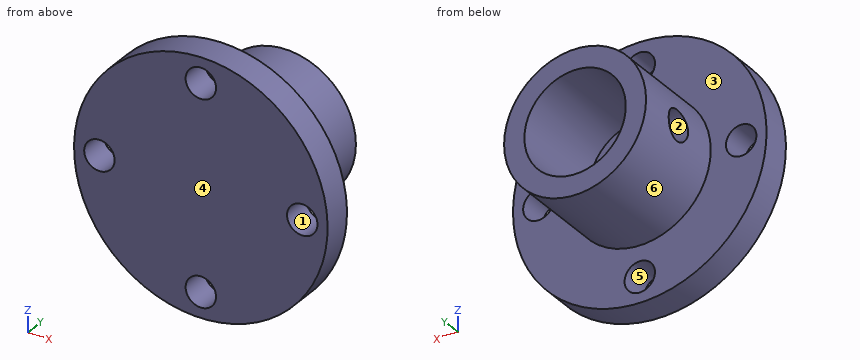
from build123d import *

# Parameters (mm, degrees)
IZIM1_R                     = 12.5
IZIM1_R_2                   = 1.5
Y_KSEKLIK_EKSTR_ZYON1_DEPTH = 3
IZIM2_R                     = 7
IZIM2_R_2                   = 5
EKSTR_ZYON_NCE1_DEPTH       = 10
IZIM3_R                     = 1.5
KES_EKSTR_ZYON1_DEPTH       = 22.943108257


with BuildPart() as part:
    # Çizim1 → Yükseklik-Ekstrüzyon1 (new body)
    with BuildSketch(Plane(origin=(0, 0, 0), x_dir=(1, 0, 0), z_dir=(0, 1, 0))):
        with Locations(Location((0, 0, 0), (0, 0, 270))):
            Circle(IZIM1_R)
        with Locations(Location((10, 0, 0), (0, 0, 270))):
            Circle(IZIM1_R_2, mode=Mode.SUBTRACT)
        with Locations(Location((0, -10, 0), (0, 0, 270))):
            Circle(IZIM1_R_2, mode=Mode.SUBTRACT)
        with Locations(Location((-10, 0, 0), (0, 0, 270))):
            Circle(IZIM1_R_2, mode=Mode.SUBTRACT)
        with Locations(Location((0, 10, 0), (0, 0, 270))):
            Circle(IZIM1_R_2, mode=Mode.SUBTRACT)
    extrude(amount=Y_KSEKLIK_EKSTR_ZYON1_DEPTH)

    # Çizim2 → Ekstrüzyon-İnce1 (add)
    with BuildSketch(Plane(origin=(0, 3, 0), x_dir=(1, 0, 0), z_dir=(0, 1, 0))):
        Circle(IZIM2_R)
        Circle(IZIM2_R_2, mode=Mode.SUBTRACT)
    extrude(amount=EKSTR_ZYON_NCE1_DEPTH)

    # Çizim3 → Kes-Ekstrüzyon1 (cut, through all)
    with BuildSketch(Plane(origin=(0, 0, 0), x_dir=(0, 0, -1), z_dir=(1, 0, 0))):
        with Locations((0, 8)):
            Circle(IZIM3_R)
    extrude(amount=-KES_EKSTR_ZYON1_DEPTH, mode=Mode.SUBTRACT)


solid = part.part
The listing builds one solid part. Answer for the finished solid, in the listing's coordinates (mm). Face numbers are marked on the shaded views. A direction names the side the tool comes from. Round coordinates to 2 decimals unless told otherwise and drop trailing zeros. Write each loop counter-clockwise with the first axis right and the second up, starting at its lowest first coordinate (ties: lowest second). Pieces come first, ordered by that corner, then holes. Notation, with made-up numbers: (-33, -1) - (-5, -1) arc R14 ccw to (-5, 23) - close; hole circle Ø6 at (11, 14). An arc over 180 degrees is marked (long way). Use one line per item in the form item = value. Start each with the question number.
Item 1: A cutting plane is placed at A-A (z = -10). Write down the section's boundary in (x, y), plus the area to 3 significant figures.
Item 2: A cutting plane is placed at B-B (x = -10). Write down the section's boundary in (y, z).
Item 3: Find the intervals of material crossed by line 1 (X direction, y = 0.8, z = 0); line 2 (Z direction, x = 0.25, y = 0.5); line 3 (X direction, y = 8.75, z = 0), in increasing order. Write a range as [from, to].
Item 4: A tool of negligible diameter and unlimited length cuts with its end or side. For the marked faces 5 and 6, from which of +Z, -Z, +X, -X, +Y, -Y can it reach the whole face along a straight path? Write none if from no direction.
Item 5: Determine the mould class of the marked faces 1, 2, 3 and 4 for opening direction Y: +Y half, -Y half, draft (parallel to the pull), parting line (faces both ways), or undercut.
Item 6: A cutting plane is placed at D-D (y = 12.25). Write down the section's boundary in (x, z), plus the area to 3 significant figures.
Item 7: Flat-ended cylindrical pins translate along their axes: pin 1 Ø4 at (x, y) = (2, 10) entering from +Z; pin 2 Ø2.5 at (y, z) = (8, 0) entering from -X; pin 3 Ø5 at (x, z) = (-10, 0) entering from +Y. Find the tip coordinate at first contact, or state that the pin passes through.
Item 8: A cutting plane is placed at C-C (x = 0.5). Write down the section's boundary in (y, z).
The answers:
q1.outline = (-7.5, 0) - (-1.5, 0) - (-1.5, 3) - (-7.5, 3) - close; (1.5, 0) - (7.5, 0) - (7.5, 3) - (1.5, 3) - close
q1.area = 36.0 mm^2
q2.outline = (0, -7.5) - (3, -7.5) - (3, -1.5) - (0, -1.5) - close; (0, 1.5) - (3, 1.5) - (3, 7.5) - (0, 7.5) - close
q3.line_1 = [-12.5, -11.5], [-8.5, 8.5], [11.5, 12.5]
q3.line_2 = [-12.5, -11.48], [-8.52, 8.52], [11.48, 12.5]
q3.line_3 = [5, 7]
q4.face_5 = +Y, -Y
q4.face_6 = +Y
q5.face_1 = draft
q5.face_2 = undercut
q5.face_3 = +Y half
q5.face_4 = -Y half
q6.outline = circle Ø14 at (0, 0); hole circle Ø10 at (0, 0)
q6.area = 75.4 mm^2
q7.pin_1 = 7
q7.pin_2 = 4.84
q7.pin_3 = 3
q8.outline = (0, -12.49) - (3, -12.49) - (3, -11.41) - (0, -11.41) - close; (0, -8.59) - (3, -8.59) - (3, -6.98) - (13, -6.98) - (13, -4.97) - (3, -4.97) - (3, 4.97) - (13, 4.97) - (13, 6.98) - (3, 6.98) - (3, 8.59) - (0, 8.59) - close; (0, 11.41) - (3, 11.41) - (3, 12.49) - (0, 12.49) - close
